Geometry: final body of the model. Coordinates: model frame, mm. A direction names the side the tool comes from. Give positions to 0.01 mm unless a question says otherwise; leave off trailing zeros. Loops run counter-clockwise (first coordinate to the right, second up) from the corner with the lowest first, then second, coordinate; pieces in that order, holes last. Notation, with made-up numbers: (48, 22.25) - (73, 22.25) arc R6 ccw to (73, 28.25) - close; hole circle Ø5 at (38, -37.5). An arc over 180 degrees is marked (long way). Answer in a Markdown table with one row per item.
from build123d import *

# Parameters (mm, degrees)
CROQUIS1_W              = 160
CROQUIS1_H              = 50
SALIENTE_EXTRUIR1_DEPTH = 10
SALIENTE_EXTRUIR2_DEPTH = 50


with BuildPart() as part:
    # Croquis1 → Saliente-Extruir1 (new body)
    with BuildSketch(Plane.XY):
        with Locations((80, 25)):
            Rectangle(CROQUIS1_W, CROQUIS1_H)
    extrude(amount=SALIENTE_EXTRUIR1_DEPTH)

    # Croquis3 → Saliente-Extruir2 (add)
    with BuildSketch(Plane.XZ):
        with BuildLine():
            Line((30, 10), (130, 10))
            ThreePointArc((130, 10), (80, 60), (30, 10))
        make_face()
    extrude(amount=-SALIENTE_EXTRUIR2_DEPTH)


solid = part.part
Q1. Material intervals for line 1 along Z through (x, y) = (80, 18.5); line 2 along Z through (x, y) = (7.5, 4.5); line 3 along X through (y, z) = (16, 32.5), sorted ascending.
Check values:
| item | result |
|---|---|
| line 1 | 0 to 60 |
| line 2 | 0 to 10 |
| line 3 | 35.35 to 124.65 |
Q2. Reachability of faces 1 (the flat face through (0, 25, 5)), 2 (the flat face through (15, 25, 10)), 3 (the flat face through (145, 25, 10)) from +Z, -Z, +X, -X, +Y, -Y: full face, straight path, thin tool, end or side. Return the list, or none.
Check values:
| item | result |
|---|---|
| face 1 | +Z, -Z, -X, +Y, -Y |
| face 2 | +Z, -X, +Y, -Y |
| face 3 | +Z, +X, +Y, -Y |
Q3. Cut plane C-C (z = 32). Output: boundary loops of the cut face in (x, y).
Check values:
| item | result |
|---|---|
| outline | (35.1, 0) - (124.9, 0) - (124.9, 50) - (35.1, 50) - close |
Q4. Cut plane B-B (x = 118). Output: boundary loops of the cut face in (y, z), and give its area (3 significant figures).
Check values:
| item | result |
|---|---|
| outline | (0, 0) - (50, 0) - (50, 42.5) - (0, 42.5) - close |
| area | 2,120 mm² |
Q5. First-contact query: pin 1 (1 mm diameter, centred on y = 35, z = 47.5, fed in from -X); pin 2 (5 mm diameter, centred on y = 26, z = 25.5, fed in from +X); pin 3 (1 mm diameter, centred on y = 20, z = 21, fed in from -X). Flat tips, straight axial feed; report the tip coordinate or a pass-through.
Check values:
| item | result |
|---|---|
| pin 1 | x = 46.37 |
| pin 2 | x = 128.28 |
| pin 3 | x = 31.11 |
Q6. Cut plane A-A (y = 22). Output: boundary loops of the cut face in (x, z), and give its area (3 significant figures).
Check values:
| item | result |
|---|---|
| outline | (0, 0) - (160, 0) - (160, 10) - (130, 10) arc R50 ccw to (30, 10) - (0, 10) - close |
| area | 5,530 mm² |
